Autodesk Inventor part; units mm, degrees
ref_plane "YZ Plane" through (0, 0, 0) normal (1, 0, 0) x (0, 1, 0)
ref_plane "XZ Plane" through (0, 0, 0) normal (0, 1, 0) x (-1, 0, 0)
ref_plane "XY Plane" through (0, 0, 0) normal (0, 0, 1) x (1, 0, 0)
sketch "Sketch1" plane through (0, 0, 0) normal (0, 1, 0) x (-1, 0, 0)
  line L0 (-15.875, 38.1) -> (15.875, 38.1)
  line L1 (25.4, 28.575) -> (25.4, -28.575)
  line L2 (15.875, -38.1) -> (-15.875, -38.1)
  line L3 (-25.4, -28.575) -> (-25.4, 28.575)
  line L4 (-25.4, 38.1) -> (25.4, -38.1) construction
  line L5 (25.4, 38.1) -> (-25.4, -38.1) construction
  arc A0 (25.4, 28.575) -> (15.875, 38.1) centre (15.875, 28.575) ccw
  arc A1 (-15.875, 38.1) -> (-25.4, 28.575) centre (-15.875, 28.575) ccw
  arc A2 (-25.4, -28.575) -> (-15.875, -38.1) centre (-15.875, -28.575) ccw
  arc A3 (15.875, -38.1) -> (25.4, -28.575) centre (15.875, -28.575) ccw
  line L6 (22.225, -28.575) -> (22.225, 28.575)
  arc A4 (22.225, 28.575) -> (15.875, 34.925) centre (15.875, 28.575) ccw
  line L7 (15.875, 34.925) -> (-15.875, 34.925)
  arc A5 (-15.875, 34.925) -> (-22.225, 28.575) centre (-15.875, 28.575) ccw
  line L8 (-22.225, 28.575) -> (-22.225, -28.575)
  arc A6 (-22.225, -28.575) -> (-15.875, -34.925) centre (-15.875, -28.575) ccw
  line L9 (-15.875, -34.925) -> (15.875, -34.925)
  arc A7 (15.875, -34.925) -> (22.225, -28.575) centre (15.875, -28.575) ccw
  point P0 (0, 0)
  dimension "d0" = 50.8
  dimension "d1" = 76.2
  dimension "d2" = 9.525
  dimension "d3" = 3.175
extrude "Extrusion1" add sketch "Sketch1" along normal blind 558.8
equation "\"d0\" = stockHeight"
equation "\"d1\" = stockWidth"
equation "\"d2\" = stockRad"
equation "\"d3\" = stockGuage"
equation "\"height\" = 203.2"
equation "\"shaftDiam\" = 6.35"
equation "\"shaftSpace\" = 1.5875"
equation "\"stageSpace\" = 2.54"
equation "\"stageAngle\" = 15deg"
equation "\"stockHeight\" = 50.8"
equation "\"stockWidth\" = 76.2"
equation "\"stockRad\" = 9.525"
equation "\"stockGuage\" = 3.175"
equation "\"groundActu\" = 304.8"
equation "\"baseWidth\" = 1066.8"
equation "\"baseDepth\" = 254"
equation "\"capThickness\" = 3.175"
equation "\"sup1Ang\" = 22.619865deg"
equation "\"sup1Len\" = 660.4"
equation "\"supVertLen\" = 955.13561"
equation "\"sup2Ang\" = 8.959949deg"
equation "\"sup2Len\" = 2079.37366"
equation "\"supSideAng\" = 19.376933deg"
equation "\"supSideLen\" = 1531.12879"
equation "\"FlangeDiam\" = 12.7"
equation "\"bearingDiam\" = 9.5504"
equation "\"FlangeDepth\" = 1.5875"
equation "\"smallFilet\" = 0.39687"
equation "\"thickness\" = 12.7"
equation "\"ringDiam\" = 96.46608"
properties part number "vertical bar" material "Aluminum 6061"
Geometry: final body of the model. Coordinates: model frame, mm. A direction names the side the tool comes from. Coordinates: 2 decimals unless noted, no trailing zeros. Order: outer loops, then holes, each group sorted by start corner. A loop starts at its lowest first (then second) coordinate and runs counter-clockwise, first axis right, second up. Notation, with made-up numbers: (61, 44.5) - (103, 44.5) arc R9 cw to (103, 61.5) - close; hole circle Ø4 at (-31, 63.25). An arc over 180 degrees is marked (long way). Use one line per item in the form item = value.
1) Set-up query: faces 1 (the face through (-22.54, 275.49, 35.38)), 2 (the face through (22.225, 275, 0)). Return all of +Z, -Z, +X, -X, +Y, -Y with unobstructed straight access to the full face (end or side cutting, diameter ignored); none if empty.
Solutions:
face_1 = +Z, -X, +Y, -Y
face_2 = +Y, -Y
2) Section C-C (z = -3). Return loops of the section in (x, y) (3 decimals), then the cut area to 3 significant figures.
Solutions:
outline = (-25.4, 0) - (-22.225, 0) - (-22.225, 558.8) - (-25.4, 558.8) - close; (22.225, 0) - (25.4, 0) - (25.4, 558.8) - (22.225, 558.8) - close
area = 3,550 mm^2
3) Section A-A (y = 365.5). Return loops of the section in (x, z) (3 decimals), then the cut area to 3 significant figures.
Solutions:
outline = (-25.4, -28.575) arc R9.525 ccw to (-15.875, -38.1) - (15.875, -38.1) arc R9.525 ccw to (25.4, -28.575) - (25.4, 28.575) arc R9.525 ccw to (15.875, 38.1) - (-15.875, 38.1) arc R9.525 ccw to (-25.4, 28.575) - close; hole (-22.225, -28.575) arc R6.35 ccw to (-15.875, -34.925) - (15.875, -34.925) arc R6.35 ccw to (22.225, -28.575) - (22.225, 28.575) arc R6.35 ccw to (15.875, 34.925) - (-15.875, 34.925) arc R6.35 ccw to (-22.225, 28.575) - close
area = 723 mm^2
4) Section B-B (x = -0.5). Return loops of the section in (y, z) (3 decimals), then the cut area to 3 significant figures.
Solutions:
outline = (0, -38.1) - (558.8, -38.1) - (558.8, -34.925) - (0, -34.925) - close; (0, 34.925) - (558.8, 34.925) - (558.8, 38.1) - (0, 38.1) - close
area = 3,550 mm^2
5) Mould query, pull axis Z, two halves, no side actions, for faces 3 (the face through (23, 558.8, -5)), 4 (the face through (-22.68, 275.49, -35.24)), 5 (the face through (0, 275, 34.925)). Classes: +Z half, -Z half, draft (parallel to the pull), parting line (faces both ways), or undercut.
Solutions:
face_3 = draft
face_4 = -Z half
face_5 = undercut
6) Ray query, L1, parallel to Z at x = -13.5, y = 384 (3 decimals); L2, parallel to X at y = 226.5, z = -20 (3 decimals); L3, parallel to Z at x = -17, y = 202.5. Return the intervals inside material, ascending.
Solutions:
L1 = -38.1 to -34.925, 34.925 to 38.1
L2 = -25.4 to -22.225, 22.225 to 25.4
L3 = -38.03 to -34.82, 34.82 to 38.03
